```python
from build123d import *

# Parameters (mm, degrees)
ESBO_O1_W                = 30
ESBO_O1_H                = 40
RESSALTO_EXTRUS_O1_DEPTH = 3
ESBO_O2_W                = 20
ESBO_O2_H                = 8
CORTE_EXTRUS_O1_DEPTH    = 26.179356624
ESBO_O3_R                = 1.2
CORTE_EXTRUS_O2_DEPTH    = 26.179356624
ESBO_O4_W                = 30
ESBO_O4_H                = 3
RESSALTO_EXTRUS_O2_DEPTH = 20
FILETE5_R                = 2.4
FILETE6_R                = 2.4
FILETE7_R                = 2.4
FILETE8_R                = 2.4


with BuildPart() as part:
    # Esboço1 → Ressalto-extrusão1 (new body)
    with BuildSketch(Plane(origin=(0, 0, 0), x_dir=(1, 0, 0), z_dir=(0, 1, 0))):
        Rectangle(ESBO_O1_W, ESBO_O1_H)
    extrude(amount=RESSALTO_EXTRUS_O1_DEPTH)

    # Esboço2 → Corte-extrusão1 (cut, through all)
    with BuildSketch(Plane(origin=(0, 3, 0), x_dir=(1, 0, 0), z_dir=(0, 1, 0))):
        with Locations((0, -11)):
            Rectangle(ESBO_O2_W, ESBO_O2_H)
    extrude(amount=-CORTE_EXTRUS_O1_DEPTH, mode=Mode.SUBTRACT)

    # Esboço3 → Corte-extrusão2 (cut, through all)
    with BuildSketch(Plane.XZ):
        with Locations(Location((-12, 17, 0), (0, 0, 270))):
            Circle(ESBO_O3_R)
        with Locations(Location((12, 17, 0), (0, 0, 270))):
            Circle(ESBO_O3_R)
        with Locations(Location((-12.5, 8, 0), (0, 0, 270))):
            Circle(ESBO_O3_R)
        with Locations(Location((12.5, 8, 0), (0, 0, 270))):
            Circle(ESBO_O3_R)
    extrude(amount=-CORTE_EXTRUS_O2_DEPTH, mode=Mode.SUBTRACT)

    # Esboço4 → Ressalto-extrusão2 (add)
    with BuildSketch(Plane.XZ):
        with Locations((0, -18.5)):
            Rectangle(ESBO_O4_W, ESBO_O4_H)
    extrude(amount=RESSALTO_EXTRUS_O2_DEPTH)

    # Filete5
    filete5_edges = [part.edges().sort_by_distance(p)[0] for p in [
        (0, 0, -17),
    ]]
    fillet(filete5_edges, radius=FILETE5_R)

    # Filete6
    filete6_edges = [part.edges().sort_by_distance(p)[0] for p in [
        (0, 3, -20),
    ]]
    fillet(filete6_edges, radius=FILETE6_R)

    # Filete7
    filete7_edges = [part.edges().sort_by_distance(p)[0] for p in [
        (15, 1.5, 20),
        (-15, 1.5, 20),
    ]]
    fillet(filete7_edges, radius=FILETE7_R)

    # Filete8
    filete8_edges = [part.edges().sort_by_distance(p)[0] for p in [
        (-15, -20, -18.5),
        (15, -20, -18.5),
    ]]
    fillet(filete8_edges, radius=FILETE8_R)


solid = part.part
```
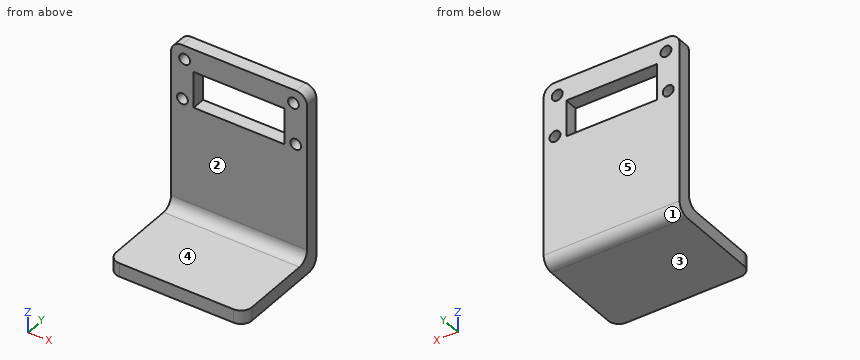
Here's how the part is built. I have some questions about the finished solid (model axes, mm). Face numbers are marked on the shaded views. A direction names the side the tool comes from. Give positions to 0.01 mm unless a question says otherwise; leave off trailing zeros. Loops run counter-clockwise (first coordinate to the right, second up) from the corner with the lowest first, then second, coordinate; pieces in that order, holes last. Notation, with made-up numbers: (54, 65) -> (80, 65) arc R33 cw to (80, 103) -> close; hole circle Ø2 at (55.5, 48). An arc over 180 degrees is marked (long way). Use one line per item in the form item = value. Start each with the question number.
1) For P1, Ø1.5, axis at x = 10.5, z = 9.5, coming from the -Y side; P2, Ø2, axis at x = -12.5, z = 8, coming from the +Y side; P3, Ø5, axis at x = -11.5, y = -11.5, coming from the +Z side, each with a flat end and sliding along its axis, tell me the tip position at first contact or that it passes through.
2) Please list where these lines run through material, in increasing order: line 1 along X through (y, z) = (0.75, 8); line 2 along X through (y, z) = (1.95, 17); line 3 along Y through (x, z) = (-7, -5).
3) Which directions (+Z, -Z, +X, -X, +Y, -Y) give clear straight access to the entire face, cutting with the end or side of a thin tool? Please do the marked faces 4 and 5.
4) Imagine slicing it at D-D (y = -4). Please give me the cut outline in (x, z), then the cut area to 3 significant figures.
5) Imagine slicing it at A-A (x = -3). Please give me the cut outline in (y, z).
6) Imagine slicing it at C-C (x = 12). Please give me the cut outline in (y, z).
7) Thinking about a two-plate mould opening in Y: for the marked faces 1, 2 and 3, which applies, +Y half, -Y half, draft (parallel to the pull), parting line (faces both ways), or undercut?
8) Imagine slicing it at B-B (z = 17). Please give me the cut outline in (x, y), then the cut area to 3 significant figures.
Check values:
q1.P1 = 0
q1.P2 = through
q1.P3 = -17
q2.line_1 = -15 to -13.7, -11.3 to -10, 10 to 11.3, 13.7 to 15
q2.line_2 = -15 to -13.2, -10.8 to 10.8, 13.2 to 15
q2.line_3 = 0 to 3
q3.face_4 = +Z, +X, -X, -Y
q3.face_5 = +Z, -Z, +X, -X, +Y
q4.outline = (-15, -20) -> (15, -20) -> (15, -17) -> (-15, -17) -> close
q4.area = 90.0 mm^2
q5.outline = (-20, -20) -> (0.6, -20) arc R2.4 ccw to (3, -17.6) -> (3, 7) -> (0, 7) -> (0, -14.6) arc R2.4 cw to (-2.4, -17) -> (-20, -17) -> close; (0, 15) -> (3, 15) -> (3, 20) -> (0, 20) -> close
q6.outline = (-20, -20) -> (0.6, -20) arc R2.4 ccw to (3, -17.6) -> (3, 6.91) -> (0, 6.91) -> (0, -14.6) arc R2.4 cw to (-2.4, -17) -> (-20, -17) -> close; (0, 9.09) -> (3, 9.09) -> (3, 15.8) -> (0, 15.8) -> close; (0, 18.2) -> (3, 18.2) -> (3, 20) -> (0, 20) -> close
q7.face_1 = +Y half
q7.face_2 = -Y half
q7.face_3 = draft
q8.outline = (-15, 0) -> (-13.2, 0) -> (-13.2, 3) -> (-15, 3) -> close; (-10.8, 0) -> (10.8, 0) -> (10.8, 3) -> (-10.8, 3) -> close; (13.2, 0) -> (15, 0) -> (15, 3) -> (13.2, 3) -> close
q8.area = 75.6 mm^2
